Autodesk Inventor part; units mm, degrees
ref_plane "Work Plane1" through (1.0409, 3.1519, 7) normal (0, 1, 0) x (-1, 0, 0)
ref_plane "YZ Plane" through (0, 0, 0) normal (1, 0, 0) x (0, 1, 0)
ref_plane "XY Plane" through (0, 0, 0) normal (0, 0, 1) x (1, 0, 0)
sketch "Sketch1" plane through (0, 0, 0) normal (0, 0, 1) x (1, 0, 0)
  circle A0 centre (1.0409, 9.1519) radius 2.25
  circle A1 centre (1.0409, 9.1519) radius 4
  point P0 (0, 0)
  dimension "d0" = 8
extrude "Extrusion1" add sketch "Sketch1" along normal blind 1 contours A0 | A1
sketch "Sketch2" plane through (1.0409, 9.1519, 1) normal (0, 0, 1) x (1, 0, 0)
  circle A0 centre (0, 0) radius 4
  point P0 (-1.0409, -9.1519)
  dimension "d3" = 8
extrude "Extrusion2" add sketch "Sketch2" along normal blind 6
sketch "Sketch3" plane through (1.0409, 9.1519, 7) normal (0, 0, 1) x (1, 0, 0)
  circle A0 centre (0, 0) radius 6
  point P0 (-1.0409, -9.1519)
  dimension "d6" = 12
extrude "Extrusion3" add sketch "Sketch3" along normal blind 1
hole "Hole1" at (1.0409, 9.1519, 8) direction (0, 0, -1) diameter 3.9 end through all
sketch "Sketch4" plane through (1.0409, 9.1519, 8) normal (0, 0, 1) x (1, 0, 0)
  line L0 (2.5, 5.4544) -> (2.5, -5.4544)
  line L1 (-2.5, -5.4544) -> (-2.5, 5.4544)
  circle A0 centre (0, 0) radius 1.95
  circle A1 centre (0, 0) radius 6
  point P0 (-1.0409, -9.1519)
  dimension "d22" = 2.5
  dimension "d23" = 2.5
extrude "Extrusion4" add sketch "Sketch4" along normal blind 6 contours L0 A1 L1 | A0
ref_plane "Work Plane1" through (1.0409, 3.1519, 7) normal (0, 1, 0) x (-1, 0, 0)
sketch "Sketch5" plane through (1.0409, 3.1519, 7) normal (0, 1, 0) x (-1, 0, 0)
  line L0 (-2.5, 1) -> (-2.5, 1)
  line L1 (-2.5, 1) -> (-2.5, 7)
  line L2 (2.5, 7) -> (-2.5, 7)
  line L3 (2.5, 1) -> (2.5, 7)
  line L4 (2.5, 1) -> (2.5, 1)
  line L5 (2.5, 1) -> (2.5, 7)
  line L6 (-2.5, 7) -> (2.5, 7)
  line L7 (-2.5, 1) -> (-2.5, 7)
  line L8 (-6, 0) -> (6, 0)
  line L9 (6, 1) -> (2.5, 1)
  arc A0 (0.9, 7) -> (2.5, 1) centre (15.8796, 7.7812) ccw
  line L10 (2.5, 7) -> (-2.5, 7)
  line L11 (0, 7) -> (0, 0)
  line L12 (4, 0) -> (-4, 0)
  line L13 (-2.5, 1) -> (-6, 1)
  arc A1 (-2.5, 1) -> (-0.9, 7) centre (-15.8796, 7.7812) ccw
  point P0 (1.0409, -7)
  dimension "d26" = 15
  dimension "d27" = 15
  dimension "d28" = 1.8
  dimension "d29" = 1.8
extrude "Extrusion5" cut sketch "Sketch5" along normal through all
chamfer "Chamfer1" distance 3 angle 45 2 edges at (1.0409, 15.1519, 14) (1.0409, 3.1519, 14)
chamfer "Chamfer2" distance 2 angle 45 1 edges at (-2.9591, 9.1519, 7)
equation "\"d23\" = d22"
equation "\"d29\" = d28"
properties part number "Arm - 608 bearing cap"
The model under review builds one solid part; all positions refer to its coordinate system, in mm. A direction names the side the tool comes from. Give positions to 0.01 mm unless a question says otherwise; leave off trailing zeros. Write each loop counter-clockwise with the first axis right and the second up, starting at its lowest first coordinate (ties: lowest second). Pieces come first, ordered by that corner, then holes. Notation, with made-up numbers: (85.5, -9) -> (137.5, -9) arc R18 cw to (137.5, 26) -> close; hole circle Ø8 at (88, 49). An arc over 180 degrees is marked (long way). Put each result on its own line as item: value.
(1) We need section B-B, the plane z = 10.5. Give the boundary of the cut face in (x, y).
Results are:
outline: (-0.46, 3.34) arc R6 ccw to (2.54, 3.34) -> (2.54, 14.96) arc R6 ccw to (-0.46, 14.96) -> close
(2) Tool access review of faces 5 (the flat face through (-3, 9, 8)), 6 (the flat face through (5, 9, 8)), 7 (the cylindrical face through (0.174, 13.057, 2.465)): name each direction out of +Z, -Z, +X, -X, +Y, -Y from which nothing blocks a thin tool from reaching the whole face with its end or side.
Results are:
face 5: +Z, -X, +Y, -Y
face 6: +Z, +X, +Y, -Y
face 7: -Z
(3) We need section C-C, the plane z = 4.75. Give the boundary of the cut face in (x, y), and give its area (3 significant figures).
Results are:
outline: circle Ø8 at (1.04, 9.15); hole circle Ø3.9 at (1.04, 9.15)
area: 38.3 mm²
(4) We need section D-D, the plane z = 12.5. Give the boundary of the cut face in (x, y).
Results are:
outline: (-0.01, 4.78) arc R4.5 ccw to (2.1, 4.78) -> (2.1, 13.53) arc R4.5 ccw to (-0.01, 13.53) -> close
(5) The part is to be moulded in two halves that separate along Y. For faces 1 (the flat face through (1, 9, 14)), 2 (the conical face through (1.06, 4.63, 12.48)), 3 (the cylindrical face through (-4.953, 8.888, 7.639)), 4 (the flat face through (1, 9, 8)), say which applies: pulls with the +Y half, pulls with the -Y half, needs draft (parallel to the pull), parting line crosses it, or undercut.
Results are:
face 1: needs draft
face 2: pulls with the -Y half
face 3: parting line crosses it
face 4: undercut
(6) We need section A-A, the plane z = 7.25. Give the boundary of the cut face in (x, y), and give its area (3 significant figures).
Results are:
outline: circle Ø12 at (1.04, 9.15); hole circle Ø3.9 at (1.04, 9.15)
area: 101 mm²
(7) To check wall thickness, follow probe 1 along X at (y, z) = (5.25, 11); probe 2 along Z at (x, y) = (1, 9.5); probe 3 along Y at (x, z) = (1.25, 5.5). State the ranges of each line that lie inside material, in increasing order. Write a range as from..to.
Results are:
probe 1: -0.32..2.4
probe 2: 8..14
probe 3: 4.66..7.21, 11.09..13.65
(8) For pin 1 Ø3 at (x, z) = (2.5, 6) entering from -Y; pin 2 Ø6 at (y, z) = (13, 7) entering from +X; pin 3 Ø6 at (y, z) = (8, 12.5) entering from +X, all flat-tipped, find the tip position at first contact; note any pin that passes through.
Results are:
pin 1: y = 3.16
pin 2: x = 6.98
pin 3: x = 2.88
